For this review, take the finished solid that the model builds, in its own axes (mm). Face numbers are marked on the shaded views. A direction names the side the tool comes from. Coordinates: 2 decimals unless noted, no trailing zeros. Write each loop counter-clockwise with the first axis right and the second up, starting at its lowest first coordinate (ties: lowest second). Pieces come first, ordered by that corner, then holes.
1) We need section A-A on z = 4. Write out the cut boundary in (x, y), then the cut area to 3 significant figures.
2) To check wall thickness, follow line 1 along X through (y, z) = (9, 1.75); line 2 along X through (y, z) = (0.5, 6.25); line 3 along Z through (x, y) = (18.75, 0.9). State the ranges of each line that lie inside material, in increasing order.
3) We need section C-C on x = -2.75. Write out the cut boundary in (y, z), then the cut area to 3 significant figures.
4) For the marked faces 3, 4 and 5, list the 3-axis set-ups (+Z, -Z, +X, -X, +Y, -Y) from which the entire face can be reached by the end or side of a thin tool; tool diameter is ignored.
5) Mouldability with a two-part tool opening along X and no side actions: class the marked faces 1 and 2 as pulls with the +X half, pulls with the -X half, needs draft (parallel to the pull), parting line crosses it, or undercut.
6) We need section B-B on y = 7.5. Write out the cut boundary in (x, z), then the cut area to 3 significant figures.
7) Insertion check: P1, Ø5, axis at x = 19.5, z = 4, coming from the +Y side; P2, Ø0.8, axis at x = -1.5, y = 0.5, coming from the +Z side; P3, Ø4, axis at y = 9, z = 8, coming from the +X side; P4, Ø2.5, axis at x = -2.75, z = 4, coming from the +Y side. Each pin has a flat end and moves straight along its axis. Give the tip position at first contact, or say it passes through.
8) We need section D-D on z = 7. Write out the cut boundary in (x, y).
from build123d import *

# Parameters (mm, degrees)
BOSS_EXTRUDE1_DEPTH = 11
SKETCH3_W           = 6.5
SKETCH3_H           = 1.5
CUT_EXTRUDE5_DEPTH  = 3
SKETCH6_R           = 1.5
CUT_EXTRUDE7_DEPTH  = 27.551836095


with BuildPart() as part:
    # Sketch1 → Boss-Extrude1 (new body)
    with BuildSketch(Plane.XY):
        with BuildLine():
            Line((0.5, 1.5), (0.5, 11.5))
            Line((0.5, 11.5), (15.5, 11.5))
            Line((15.5, 11.5), (15.5, 1.5))
            Line((15.5, 1.5), (22, 1.5))
            Line((22, 1.5), (22, 0))
            Line((22, 0), (14, 0))
            Line((14, 0), (14, 9))
            ThreePointArc((14, 9), (13.707106781, 9.707106781), (13, 10))
            Line((13, 10), (3, 10))
            ThreePointArc((3, 10), (2.292893219, 9.707106781), (2, 9))
            Line((2, 9), (2, 0))
            Line((2, 0), (-6, 0))
            Line((-6, 0), (-6, 1.5))
            Line((-6, 1.5), (0.5, 1.5))
        make_face()
    extrude(amount=BOSS_EXTRUDE1_DEPTH)

    # Sketch3 → Cut-Extrude5 (cut)
    with BuildSketch(Plane.XY.offset(11)):
        with Locations((-2.75, 0.75)):
            Rectangle(SKETCH3_W, SKETCH3_H)
        with Locations((18.75, 0.75)):
            Rectangle(SKETCH3_W, SKETCH3_H)
    extrude(amount=-CUT_EXTRUDE5_DEPTH, mode=Mode.SUBTRACT)

    # Sketch6 → Cut-Extrude7 (cut, through all)
    with BuildSketch(Plane(origin=(0, 1.5, 0), x_dir=(1, 0, 0), z_dir=(0, 1, 0))):
        with Locations(Location((-2.75, -4, 0), (0, 0, 180))):
            Circle(SKETCH6_R)
        with Locations((18.75, -4)):
            Circle(SKETCH6_R)
        Polygon((-6, -1.5), (-4.5, 0), (-6, 0), align=None)
        Polygon((20.5, 0), (22, 0), (22, -1.5), align=None)
        Polygon((22, -6.5), (20.5, -8), (22, -8), align=None)
        Polygon((-4.5, -8), (-6, -8), (-6, -6.5), align=None)
    extrude(amount=-CUT_EXTRUDE7_DEPTH, mode=Mode.SUBTRACT)


solid = part.part
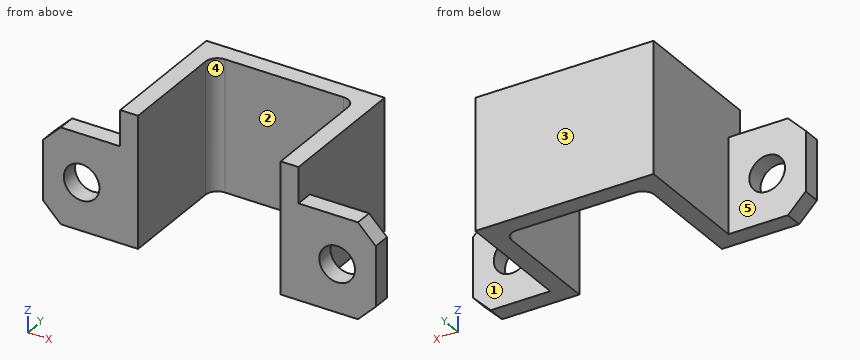
Result:
1. outline: (-6, 0) - (-4.25, 0) - (-4.25, 1.5) - (-6, 1.5) - close; (-1.25, 0) - (2, 0) - (2, 9) arc R1 cw to (3, 10) - (13, 10) arc R1 cw to (14, 9) - (14, 0) - (17.25, 0) - (17.25, 1.5) - (15.5, 1.5) - (15.5, 11.5) - (0.5, 11.5) - (0.5, 1.5) - (-1.25, 1.5) - close; (20.25, 0) - (22, 0) - (22, 1.5) - (20.25, 1.5) - close
1. area: 63.4 mm2
2. line 1: x = 0.5 to 2, 14 to 15.5
2. line 2: x = -6 to 2, 14 to 22
2. line 3: z = 0 to 2.5, 5.5 to 8
3. outline: (0, 0) - (1.5, 0) - (1.5, 2.5) - (0, 2.5) - close; (0, 5.5) - (1.5, 5.5) - (1.5, 8) - (0, 8) - close
3. area: 7.50 mm2
4. face 3: +Z, -Z, +X, -X, +Y
4. face 4: +Z, -Z, -Y
4. face 5: +Z, -Z, -X, +Y
5. face 1: needs draft
5. face 2: undercut
6. outline: (0.5, 0) - (2, 0) - (2, 11) - (0.5, 11) - close; (14, 0) - (15.5, 0) - (15.5, 11) - (14, 11) - close
6. area: 33.0 mm2
7. P1: stops at y = 1.5
7. P2: stops at z = 8
7. P3: stops at x = 15.5
7. P4: passes through
8. outline: (-5.5, 0) - (2, 0) - (2, 9) arc R1 cw to (3, 10) - (13, 10) arc R1 cw to (14, 9) - (14, 0) - (21.5, 0) - (21.5, 1.5) - (15.5, 1.5) - (15.5, 11.5) - (0.5, 11.5) - (0.5, 1.5) - (-5.5, 1.5) - close
